Build history of the part. All positions in model axes, mm. Face numbers are marked on the shaded views. A direction names the side the tool comes from. Round coordinates to 2 decimals unless told otherwise and drop trailing zeros. Loops run counter-clockwise (first coordinate to the right, second up) from the corner with the lowest first, then second, coordinate; pieces in that order, holes last. Notation, with made-up numbers: (49, -26.5) - (65, -26.5) arc R11 cw to (65, -14.5) - close; hole circle Ø3 at (29, -31). An arc over 180 degrees is marked (long way). Use a Markdown table: item, result.
from build123d import *

# Parameters (mm, degrees)
BOSS_EXTRUDE1_DEPTH                                 = 5
FILLET1_R                                           = 2
FILLET2_R                                           = 2.5
CUT_EXTRUDE2_REACH                                  = 7
CSK_FOR_M2_COUNTERSUNK_FLAT_HEAD_SCREW1_D           = 2.2
CSK_FOR_M2_COUNTERSUNK_FLAT_HEAD_SCREW1_DEPTH       = 5
CSK_FOR_M2_COUNTERSUNK_FLAT_HEAD_SCREW1_CSINK_D     = 4.9
CSK_FOR_M2_COUNTERSUNK_FLAT_HEAD_SCREW1_CSINK_ANGLE = 90
M2_TAPPED_HOLE1_D                                   = 1.6
M2_TAPPED_HOLE1_DEPTH                               = 5
SKETCH9_W                                           = 25.2
SKETCH9_H                                           = 12.5
CUT_EXTRUDE3_DEPTH                                  = 1.25
CUT_EXTRUDE4_DEPTH                                  = 1.25


with BuildPart() as part:
    # Sketch1 → Boss-Extrude1 (new body)
    with BuildSketch(Plane(origin=(0, 0, 0), x_dir=(1, 0, 0), z_dir=(0, 1, 0))):
        Polygon((0, 35), (0, 10.25), (4.1, 10.25), (4.1, -10.25), (0, -10.25), (0, -35), (40, -35), (40, -17.5), (15, -17.5), (15, 17.5), (40, 17.5), (40, 35), align=None)
    extrude(amount=BOSS_EXTRUDE1_DEPTH)

    # Fillet1
    fillet1_edges = [part.edges().sort_by_distance(p)[0] for p in [
        (15, 2.5, -17.5),
        (15, 2.5, 17.5),
    ]]
    fillet(fillet1_edges, radius=FILLET1_R)

    # Fillet2
    fillet2_edges = [part.edges().sort_by_distance(p)[0] for p in [
        (0, 2.5, -35),
        (40, 2.5, -35),
        (40, 2.5, 35),
        (0, 2.5, 35),
    ]]
    fillet(fillet2_edges, radius=FILLET2_R)

    # Sketch3 → Cut-Extrude2 (cut, up to next)
    with BuildSketch(Plane(origin=(0, 5, 0), x_dir=(1, 0, 0), z_dir=(0, 1, 0)), mode=Mode.PRIVATE) as cut_extrude2_sk1:
        with BuildLine():
            Line((4.1, 10.25), (4.35, 10.25))
            ThreePointArc((4.35, 10.25), (5.35, 9.25), (4.35, 8.25))
            Line((4.35, 8.25), (4.1, 8.25))
            Line((4.1, 8.25), (4.1, 10.25))
        make_face()
    cut_extrude2_tool1 = extrude(cut_extrude2_sk1.sketch, amount=-CUT_EXTRUDE2_REACH, mode=Mode.PRIVATE) & part.part
    add(cut_extrude2_tool1.solids().sort_by_distance((4.641756, 5, -9.25))[0], mode=Mode.SUBTRACT)
    # Sketch3 → Cut-Extrude2 (cut, up to next)
    with BuildSketch(Plane(origin=(0, 5, 0), x_dir=(1, 0, 0), z_dir=(0, 1, 0)), mode=Mode.PRIVATE) as cut_extrude2_sk2:
        with BuildLine():
            Line((4.1, -10.25), (4.1, -8.25))
            Line((4.1, -8.25), (4.35, -8.25))
            ThreePointArc((4.35, -8.25), (5.35, -9.25), (4.35, -10.25))
            Line((4.35, -10.25), (4.1, -10.25))
        make_face()
    cut_extrude2_tool2 = extrude(cut_extrude2_sk2.sketch, amount=-CUT_EXTRUDE2_REACH, mode=Mode.PRIVATE) & part.part
    add(cut_extrude2_tool2.solids().sort_by_distance((4.641756, 5, 9.25))[0], mode=Mode.SUBTRACT)

    # CSK for M2 Countersunk Flat Head Screw1
    with Locations(Plane(origin=(0, 5, 0), x_dir=(1, 0, 0), z_dir=(0, 1, 0))):
        with Locations((4, 30), (4, 15), (4, -15), (4, -30)):
            csk_for_m2_countersunk_flat_head_screw1 = CounterSinkHole(CSK_FOR_M2_COUNTERSUNK_FLAT_HEAD_SCREW1_D / 2, CSK_FOR_M2_COUNTERSUNK_FLAT_HEAD_SCREW1_CSINK_D / 2, depth=CSK_FOR_M2_COUNTERSUNK_FLAT_HEAD_SCREW1_DEPTH, counter_sink_angle=CSK_FOR_M2_COUNTERSUNK_FLAT_HEAD_SCREW1_CSINK_ANGLE)

    # M2 Tapped Hole1
    with Locations(Plane(origin=(0, 5, 0), x_dir=(1, 0, 0), z_dir=(0, 1, 0))):
        with Locations((12.5, -25), (12.5, 25)):
            Hole(M2_TAPPED_HOLE1_D / 2, depth=M2_TAPPED_HOLE1_DEPTH)

    # Sketch9 → Cut-Extrude3 (cut)
    with BuildSketch(Plane(origin=(0, 5, 0), x_dir=(1, 0, 0), z_dir=(0, 1, 0))):
        with Locations((27.4, 26.25)):
            Rectangle(SKETCH9_W, SKETCH9_H)
        with Locations((27.4, -26.25)):
            Rectangle(SKETCH9_W, SKETCH9_H)
    extrude(amount=-CUT_EXTRUDE3_DEPTH, mode=Mode.SUBTRACT)

    # Sketch10 → Cut-Extrude4 (cut)
    with BuildSketch(Plane(origin=(0, 5, 0), x_dir=(1, 0, 0), z_dir=(0, 1, 0))):
        with BuildLine():
            Line((14.8, 22), (14.8, 20))
            ThreePointArc((14.8, 20), (13.8, 21), (14.8, 22))
        make_face()
        with BuildLine():
            Line((14.8, 30.5), (14.8, 32.5))
            ThreePointArc((14.8, 32.5), (13.8, 31.5), (14.8, 30.5))
        make_face()
    cut_extrude4 = extrude(amount=-CUT_EXTRUDE4_DEPTH, mode=Mode.SUBTRACT)

    # Mirror1: CSK for M2 Countersunk Flat Head Screw1 across plane
    add(csk_for_m2_countersunk_flat_head_screw1.mirror(Plane(origin=(0, 2.5, 0), x_dir=(0, 0, 1), z_dir=(0, -1, 0))), mode=Mode.SUBTRACT)

    # Mirror2: Cut-Extrude4 across plane
    add(cut_extrude4.mirror(Plane.XY), mode=Mode.SUBTRACT)


solid = part.part
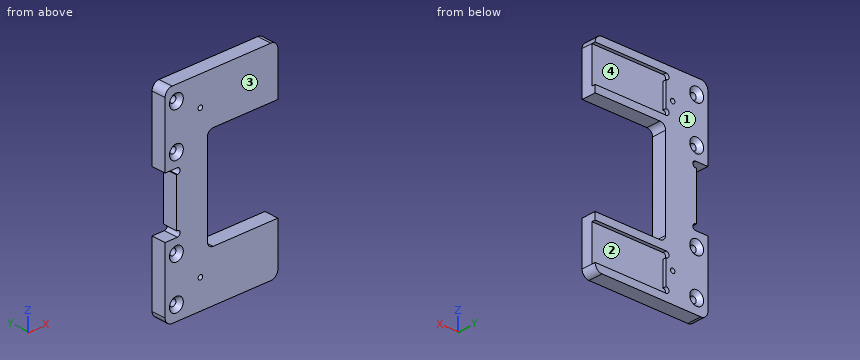
Q1. Cut at A-A, the plane x = 18. List the corners of the cut face in (y, z), plus the area to 3 significant figures.
Results found:
| item | result |
|---|---|
| outline | (0, -35) - (5, -35) - (5, -32.5) - (3.75, -32.5) - (3.75, -20) - (5, -20) - (5, -17.5) - (0, -17.5) - close; (0, 17.5) - (5, 17.5) - (5, 20) - (3.75, 20) - (3.75, 32.5) - (5, 32.5) - (5, 35) - (0, 35) - close |
| area | 144 mm2 |
Q2. Drop flat-ended pins along their axis: pin 1 (3 mm diameter, centred on x = 4, z = 15, fed in from +Y); pin 2 (1.8 mm diameter, centred on x = 4, z = -15, fed in from -Y); pin 3 (2.5 mm diameter, centred on y = 3, z = 1.5, fed in from +X); pin 4 (3.5 mm diameter, centred on x = 4, z = -30, fed in from +Y). Give the stop position or say it passes through.
Results found:
| item | result |
|---|---|
| pin 1 | stops at y = 4.05 |
| pin 2 | passes through |
| pin 3 | stops at x = 15 |
| pin 4 | stops at y = 4.3 |
Q3. Probe line 1 (Z direction, x = 4, y = 2.35); line 2 (Z direction, x = 12.5, y = 2.25); line 3 (X direction, y = 1.15, z = -25). List the from-to ranges inside material, lowest first.
Results found:
| item | result |
|---|---|
| line 1 | z = -35 to -31.1, -28.9 to -16.1, -13.9 to -10.25, 10.25 to 13.9, 16.1 to 28.9, 31.1 to 35 |
| line 2 | z = -35 to -25.8, -24.2 to 24.2, 25.8 to 35 |
| line 3 | x = 0 to 11.7, 13.3 to 40 |
Q4. Cut at D-D, the plane z = -21. List the corners of the cut face in (x, y), plus the area to 3 significant figures.
Results found:
| item | result |
|---|---|
| outline | (0, 0) - (40, 0) - (40, 3.75) - (13.8, 3.75) - (13.8, 5) - (0, 5) - close |
| area | 167 mm2 |
Q5. Pull direction Z, two halves, no side cores. Call the marked faces 3 and 4: pulls with the +Z half, pulls with the -Z half, needs draft (parallel to the pull), parting line crosses it, or undercut.
Results found:
| item | result |
|---|---|
| face 3 | needs draft |
| face 4 | undercut |
Q6. Cut at B-B, the plane z = 25. List the corners of the cut face in (x, y), plus the area to 4 significant figures.
Results found:
| item | result |
|---|---|
| outline | (0, 0) - (11.7, 0) - (11.7, 5) - (0, 5) - close; (13.3, 0) - (40, 0) - (40, 3.75) - (14.8, 3.75) - (14.8, 5) - (13.3, 5) - close |
| area | 160.5 mm2 |
Q7. Which spindle directions (+Z, -Z, +X, -X, +Y, -Y) get a long thin tool onto all of the face, cutting with end or side? Do the marked faces 1 and 2. Say none if no direction does.
Results found:
| item | result |
|---|---|
| face 1 | +Z, -Z, +X, -X, +Y |
| face 2 | +X, +Y |
Q8. Cut at C-C, the plane y = 3. List the corners of the cut face in (x, z), plus the area to 3 significant figures.
Results found:
| item | result |
|---|---|
| outline | (0, -32.5) arc R2.5 ccw to (2.5, -35) - (37.5, -35) arc R2.5 ccw to (40, -32.5) - (40, -17.5) - (17, -17.5) arc R2 cw to (15, -15.5) - (15, 15.5) arc R2 cw to (17, 17.5) - (40, 17.5) - (40, 32.5) arc R2.5 ccw to (37.5, 35) - (2.5, 35) arc R2.5 ccw to (0, 32.5) - (0, 10.25) - (4.35, 10.25) arc R1 cw to (4.35, 8.25) - (4.1, 8.25) - (4.1, -8.25) - (4.35, -8.25) arc R1 cw to (4.35, -10.25) - (0, -10.25) - close; hole circle Ø2.2 at (4, -30); hole circle Ø2.2 at (4, -15); hole circle Ø2.2 at (4, 15); hole circle Ø2.2 at (4, 30); hole circle Ø1.6 at (12.5, -25); hole circle Ø1.6 at (12.5, 25) |
| area | 1,810 mm2 |
